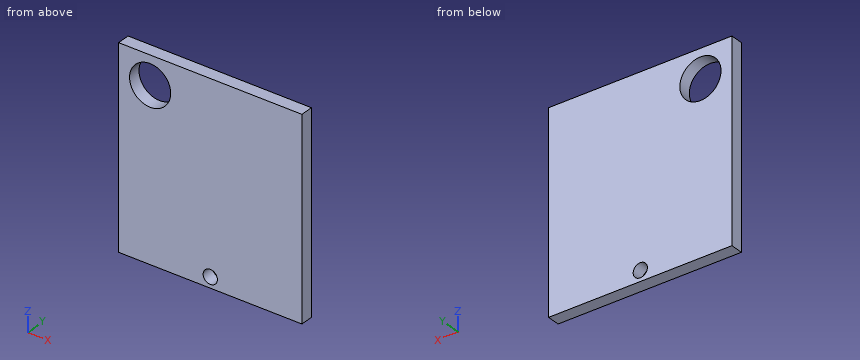
```python
from build123d import *

# Parameters (mm, degrees)
ESQUISSE2_W             = 57.9
ESQUISSE2_H             = 62.35
BOSS_EXTRU_1_DEPTH      = 4
ESQUISSE3_R             = 6.5
ENL_V_MAT_EXTRU_1_DEPTH = 51.389483469
ESQUISSE4_R             = 2.25
ENL_V_MAT_EXTRU_2_DEPTH = 10


with BuildPart() as part:
    # Esquisse2 → Boss.-Extru.1 (new body)
    with BuildSketch(Plane(origin=(0, 0, 0), x_dir=(1, 0, 0), z_dir=(0, 1, 0))):
        with Locations((0, -9.873721591)):
            Rectangle(ESQUISSE2_W, ESQUISSE2_H)
    extrude(amount=BOSS_EXTRU_1_DEPTH)

    # Esquisse3 → Enlèv. mat.-Extru.1 (cut, through all)
    with BuildSketch(Plane.XZ):
        with Locations(Location((-19, 32, 0), (0, 0, 270))):
            Circle(ESQUISSE3_R)
    extrude(amount=-ENL_V_MAT_EXTRU_1_DEPTH, mode=Mode.SUBTRACT)

    # Esquisse4 → Enlèv. mat.-Extru.2 (cut)
    with BuildSketch(Plane(origin=(0, 4, 0), x_dir=(1, 0, 0), z_dir=(0, 1, 0))):
        with Locations(Location((0, 17.951278409, 0), (0, 0, 270))):
            Circle(ESQUISSE4_R)
    extrude(amount=-ENL_V_MAT_EXTRU_2_DEPTH, mode=Mode.SUBTRACT)


solid = part.part
```
Geometry check sheet. Reference: the model listing, model coordinates, mm. Coordinates: 2 decimals unless noted, no trailing zeros. Loops run counter-clockwise (first coordinate to the right, second up) from the corner with the lowest first, then second, coordinate; pieces in that order, holes last. Notation, with made-up numbers: (-3, -4) - (29, -4) arc R33 ccw to (29, 29) - close; hole circle Ø7 at (7.25, 6.25). An arc over 180 degrees is marked (long way). One line per item, written item: value. Start each with the question number.
(1) Cross-section at C-C on y = 1.3. Enter the section's corners in (x, z), plus the area to 3 significant figures.
(2) Cross-section at A-A on x = -19. Enter the section's corners in (y, z).
(3) Material ranges on line 1 (X direction, y = 1.6, z = 32); line 2 (Z direction, x = 0.5, y = 1.55); line 3 (X direction, y = 0.7, z = -16.5), recorded low to high. Write a range as [from, to].
(4) Cross-section at B-B on z = 32. Enter the section's corners in (x, y), plus the area to 3 significant figures.
Results below:
1. outline: (-28.95, -21.3) - (28.95, -21.3) - (28.95, 41.05) - (-28.95, 41.05) - close; hole circle Ø13 at (-19, 32); hole circle Ø4.5 at (0, -17.95)
1. area: 3,460 mm2
2. outline: (0, -21.3) - (4, -21.3) - (4, 25.5) - (0, 25.5) - close; (0, 38.5) - (4, 38.5) - (4, 41.05) - (0, 41.05) - close
3. line 1: x = [-28.95, -25.5], [-12.5, 28.95]
3. line 2: z = [-21.3, -20.15], [-15.76, 41.05]
3. line 3: x = [-28.95, -1.72], [1.72, 28.95]
4. outline: (-28.95, 0) - (-25.5, 0) - (-25.5, 4) - (-28.95, 4) - close; (-12.5, 0) - (28.95, 0) - (28.95, 4) - (-12.5, 4) - close
4. area: 180 mm2
